Autodesk Fusion 360 part; units mm, degrees
sketch "Sketch1" plane through (0, 0, 0) normal (0, 0, 1) x (1, 0, 0)
  circle A0 centre (-57, 0.002) radius 11
  circle A1 centre (57, 0.0006) radius 11
  line L0 (57.0004, 32.0006) -> (-56.9996, 32.002)
  line L1 (-57.0004, -31.998) -> (56.9996, -31.9994)
  line L2 (-32, 32.0017) -> (-32.0007, -31.9983)
  line L3 (32.0004, 32.0009) -> (31.9996, -31.9991)
  line L4 (-19.0007, -31.9985) -> (-19.0002, 19.0015)
  line L5 (18.9996, -31.9989) -> (19.0002, 19.0011)
  line L6 (-19.0004, 19.0015) -> (19.0002, 19.0011)
  arc A2 (-56.9996, 32.002) -> (-57.0004, -31.998) centre (-57, 0.002) ccw
  arc A3 (56.9996, -31.9994) -> (57.0004, 32.0006) centre (57, 0.0006) ccw
  dimension "d1" = 22
  dimension "d2" = 57
  dimension "d3" = 22
  dimension "d4" = 57
  dimension "d7" = 114
  dimension "d8" = 64
  dimension "d9" = 32
  dimension "d10" = 32
  dimension "d13" = 51
extrude "Extrude2" add sketch "Sketch1" along normal blind 19 contours L0 L1 L3 A3 makes body 1
extrude "Extrude1" add sketch "Sketch1" along normal blind 19 separate body contours L0 L1 L2 A2 makes body 2
extrude "Extrude3" add sketch "Sketch1" along normal blind 13 separate body contours L1 L4 L5 L6 makes body 3
extrude "Extrude4" add sketch "Sketch1" along normal blind 64 contours L0 L1 L2 L3 L4 L5 L6 bodies 1 2 3
sketch "Sketch3" plane through (19, -0.0002, 0) normal (-1, 0, 0) x (0, -1, 0)
  line L0 (-19.0013, 13) -> (31.9987, 13)
  line L1 (31.9987, 13) -> (31.9987, 64)
  line L2 (31.9987, 64) -> (-19.0013, 64)
  line L3 (-19.0013, 64) -> (-19.0013, 13)
  line L4 (-19.0013, 64) -> (31.9987, 13)
  line L5 (-19.0013, 64) -> (-19.0013, 13)
  line L6 (31.9987, 13) -> (-19.0013, 13)
extrude "Extrude5" add sketch "Sketch3" along normal blind 38 contours L0 L3 L4 L5 L6 bodies 1
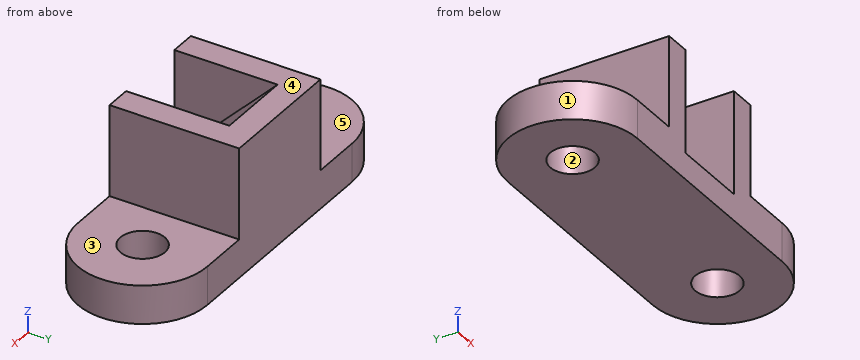
Geometry: final body of the model. Coordinates: model frame, mm. Face numbers are marked on the shaded views. A direction names the side the tool comes from. Round coordinates to 2 decimals unless told otherwise and drop trailing zeros. Order: outer loops, then holes, each group sorted by start corner. A loop starts at its lowest first (then second) coordinate and runs counter-clockwise, first axis right, second up. Notation, with made-up numbers: (42.5, -32.5) - (69.5, -32.5) arc R9 ccw to (69.5, -23.5) - close; hole circle Ø6 at (59.25, 31.25). An arc over 180 degrees is marked (long way). Write item = value, one per line. Start each with the question number.
Q1. Access query for the marked faces 4 and 5. Directions: +Z, -Z, +X, -X, +Y, -Y. A direction counts if a zero-diameter tool reaches every point of the face in a straight line with its end or side. Return the directions, or none.
Q2. Cut plane C-C on y = 2. Give the number of separate pieces and of enclosed holes in the cut face, and give its area (3 significant figures).
Q3. Ray query, line 1 (X direction, y = -2, z = 49); line 2 (Y direction, x = 57, z = 15); line 3 (Z direction, x = -42.5, y = -21). Return the intervals inside material, ascending. Write a range as from..to.
Q4. Pin query (flat end, axial travel): pin 1 (13.5 mm diameter, centred on y = 5, z = 31, fed in from +X); pin 2 (13.5 mm diameter, centred on y = 3.5, z = 41.5, fed in from -X); pin 3 (1 mm diameter, centred on x = 15.5, z = 27, fed in from -Y). Return the tip coordinate at first contact, or that it passes through.
Q5. Pull-direction query (Y, two-part tool) for the marked faces 1, 2 and 3; classes: +Y half, -Y half, draft (parallel to the pull), parting line (faces both ways), or undercut.
Q6. Cut plane B-B on x = 63.5. Return the cut outline in (y, z).
Outcome:
q1.face_4 = +Z, +X, -X, +Y, -Y
q1.face_5 = +Z, -X, +Y, -Y
q2.separate_pieces = 3
q2.enclosed_holes = 0
q2.area = 4,790 mm^2
q3.line_1 = -32..-19, 19..32
q3.line_2 = -32..-11, 11..32
q3.line_3 = 0..19
q4.pin_1 = 32
q4.pin_2 = -32
q4.pin_3 = -18.5
q5.face_1 = parting line
q5.face_2 = undercut
q5.face_3 = draft
q6.outline = (-31.33, 0) - (-8.87, 0) - (-8.87, 19) - (-31.33, 19) - close; (8.87, 0) - (31.33, 0) - (31.33, 19) - (8.87, 19) - close
